from build123d import *

# Parameters (mm, degrees)
SKETCH_1_R      = 8
SKETCH_1_R_2    = 1.6
EXTRUDE_1_DEPTH = 5
FILLET_1_R      = 10


with BuildPart() as part:
    # ｽｹｯﾁ1 → ﾎﾞｽ - 押し出し1 (new body)
    with BuildSketch(Plane.XY):
        Polygon((0, 0), (0, 10), (0, 30), (30, 30), (70, 10), (70, 0), align=None)
        with Locations((15, 15)):
            Circle(SKETCH_1_R, mode=Mode.SUBTRACT)
        with Locations((5, 5)):
            Circle(SKETCH_1_R_2, mode=Mode.SUBTRACT)
        with Locations((65, 5)):
            Circle(SKETCH_1_R_2, mode=Mode.SUBTRACT)
    extrude(amount=EXTRUDE_1_DEPTH)

    # ﾌｨﾚｯﾄ1
    fillet_1_edges = [part.edges().sort_by_distance(p)[0] for p in [
        (0, 30, 2.5),
        (30, 30, 2.5),
    ]]
    fillet(fillet_1_edges, radius=FILLET_1_R)


solid = part.part
Here's how the part is built. I have some questions about the finished solid (model axes, mm). Coordinates: 2 decimals unless noted, no trailing zeros. Write each loop counter-clockwise with the first axis right and the second up, starting at its lowest first coordinate (ties: lowest second). Pieces come first, ordered by that corner, then holes. Notation, with made-up numbers: (52, 49) - (80, 49) arc R16 cw to (80, 60) - close; hole circle Ø2 at (53.5, -19). An arc over 180 degrees is marked (long way). Use one line per item in the form item = value.
1) Suppose I cut it at D-D, the plane z = 3.75. Write out the boundary of the cut face in (x, y).
Solved:
outline = (0, 0) - (70, 0) - (70, 10) - (32.11, 28.94) arc R10 ccw to (27.64, 30) - (10, 30) arc R10 ccw to (0, 20) - close; hole circle Ø3.2 at (5, 5); hole circle Ø16 at (15, 15); hole circle Ø3.2 at (65, 5)
2) Suppose I cut it at A-A, the plane y = 5. Write out the boundary of the cut face in (x, z).
Solved:
outline = (0, 0) - (3.4, 0) - (3.4, 5) - (0, 5) - close; (6.6, 0) - (63.4, 0) - (63.4, 5) - (6.6, 5) - close; (66.6, 0) - (70, 0) - (70, 5) - (66.6, 5) - close
3) I need wall thicknesses on line 1 (X direction, y = 6, z = 1.5); line 2 (X direction, y = 8.75, z = 3.3); line 3 (Y direction, x = 15, z = 2.8). Which ranges of each line are inside material? Lowest first, please.
Solved:
line_1 = 0 to 3.75, 6.25 to 63.75, 66.25 to 70
line_2 = 0 to 10.01, 19.99 to 70
line_3 = 0 to 7, 23 to 30
4) Suppose I cut it at B-B, the plane x = 15. Write out the boundary of the cut face in (y, z).
Solved:
outline = (0, 0) - (7, 0) - (7, 5) - (0, 5) - close; (23, 0) - (30, 0) - (30, 5) - (23, 5) - close
5) Suppose I cut it at C-C, the plane y = 15. Write out the boundary of the cut face in (x, z), plus the area to 3 significant figures.
Solved:
outline = (0, 0) - (7, 0) - (7, 5) - (0, 5) - close; (23, 0) - (60, 0) - (60, 5) - (23, 5) - close
area = 220 mm2
6) Thinking about a two-plate mould opening in Y: for faces 1 (the flat face through (19, 30, 2)), 2 (the cylindrical face through (13.27, 7.19, 2.46)), 3 (the flat face through (35, 0, 2)), 4 (the flat face through (70, 5, 2)), which applies, released by +Y, released by -Y, zero draft, split by the parting line, or undercut?
Solved:
face_1 = released by +Y
face_2 = undercut
face_3 = released by -Y
face_4 = zero draft
